Could you check a few things on this model? Use its own coordinates, in mm. Give positions to 0.01 mm unless a question says otherwise; leave off trailing zeros. Loops run counter-clockwise (first coordinate to the right, second up) from the corner with the lowest first, then second, coordinate; pieces in that order, holes last. Notation, with made-up numbers: M 49,-33 L 91,-33 A15 ccw 91,-27 Z; hole C -34.5,87 d11. An arc over 180 degrees is marked long. Return JSON: item names as keys, results as strings. Group by question number.
1. For pin 1 (1.5 mm diameter, centred on y = -433.5, z = -3, fed in from -X); pin 2 (2.5 mm diameter, centred on y = -432, z = -3, fed in from +X); pin 3 (1.5 mm diameter, centred on x = 51.5, z = -2.5, fed in from -Y), each with a flat end and sliding along its axis, tell me the tip position at first contact or that it passes through.
2. Please list where these lines run through material, in increasing order: line 1 (X direction, y = -433, z = -1.25); line 2 (Y direction, x = 346.5, z = -4.5); line 3 (X direction, y = -429.5, z = -3.1).
3. If we section it at B-B (x = 115.5): Write out the boundary of the cut face in (y, z), plus the area to 3 significant figures.
```python
from build123d import *

# Parameters (mm, degrees)
BOSS_EXTRUDE1_DEPTH = 5


with BuildPart() as part:
    # Sketch1 → Boss-Extrude1 (new body)
    with BuildSketch(Plane.XY):
        Polygon((440.000271395, -430), (440.000271395, -422.5), (445, -422.5), (445, -407.5), (440.000271395, -407.5), (440.000271395, -400), (9.999728605, -400), (9.999728605, -407.5), (5, -407.5), (5, -422.5), (9.999728605, -422.5), (9.999728605, -430), (70, -430), (70, -435), (100, -435), (100, -430), (140, -430), (140, -435), (170, -435), (170, -430), (210, -430), (210, -435), (240, -435), (240, -430), (280, -430), (280, -435), (310, -435), (310, -430), (350, -430), (350, -435), (380, -435), (380, -430), align=None)
    extrude(amount=-BOSS_EXTRUDE1_DEPTH)


solid = part.part
```
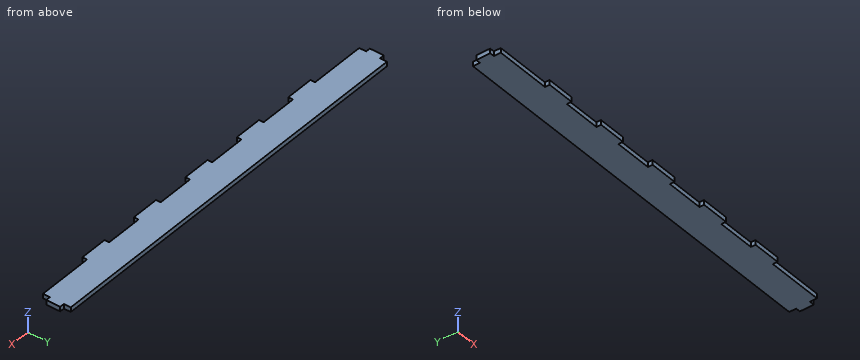
Answer:
{
 "1": {"pin 1": "stops at x = 70", "pin 2": "stops at x = 380", "pin 3": "stops at y = -430"},
 "2": {"line 1": "x = 70 to 100, 140 to 170, 210 to 240, 280 to 310, 350 to 380", "line 2": "y = -430 to -400", "line 3": "x = 10 to 440"},
 "3": {"outline": "M -430,-5 L -400,-5 L -400,0 L -430,0 Z", "area": "150 mm²"}
}
